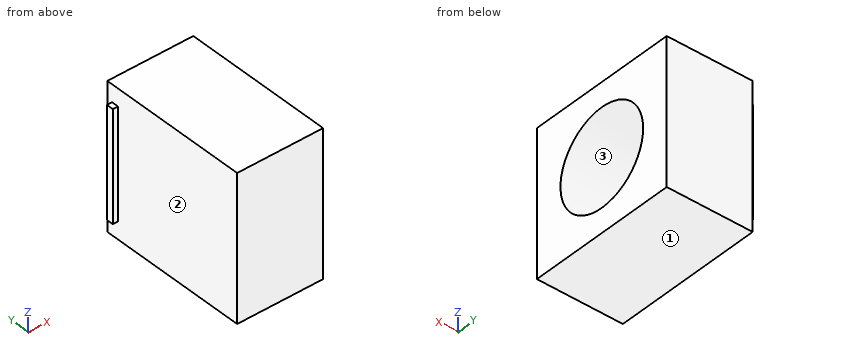
from build123d import *

# Parameters (mm, degrees)
F0_W     = 79.375
F0_H     = 133.35
F1_DEPTH = 139.7
F2_R     = 44.45
F3_DEPTH = 76.2
F4_W     = 6.35
F4_H     = 101.6
F5_DEPTH = 44.45


# Not quite as in the source:
# - a feature names something its author has since deleted; it is built from what else it names


with BuildPart() as f1:
    # F0 (on Front) → F1 (new body)
    with BuildSketch(Plane.XZ):
        Rectangle(F0_W, F0_H)
    extrude(amount=F1_DEPTH)

    # F2 (on face) → F3 (cut)
    with BuildSketch(Plane.YZ.offset(39.6875)):
        with Locations((-69.85, 0)):
            Circle(F2_R)
    extrude(amount=-F3_DEPTH, mode=Mode.SUBTRACT)

    # F4 (on Right) → F5 (join)
    with BuildSketch(Plane.YZ):
        with Locations((-8.2414448261, 0)):
            Rectangle(F4_W, F4_H)
    extrude(amount=-F5_DEPTH)


solid = f1.part
Design review of the part built by this model. Coordinates are the model's own, in mm. Face numbers are marked on the shaded views. Round coordinates to 2 decimals unless told otherwise and drop trailing zeros. Write each loop counter-clockwise with the first axis right and the second up, starting at its lowest first coordinate (ties: lowest second). Pieces come first, ordered by that corner, then holes. Notation, with made-up numbers: (82, -29.5) -> (88, -29.5) arc R5 ccw to (88, -21.5) -> close; hole circle Ø6 at (34, -15.5). An arc over 180 degrees is marked (long way). One line per item, written item: value. Start each with the question number.
Q1. Add section C-C (x = 4.5). Give the boundary of the cut face in (y, z) (3 decimals), then the cut area to 3 significant figures.
Q2. The part is to be moulded in two halves that separate along Z. For the marked faces 1, 2 and 3, say which applies: pulls with the +Z half, pulls with the -Z half, needs draft (parallel to the pull), parting line crosses it, or undercut.
Q3. Add section D-D (y = -92.5). Give the boundary of the cut face in (x, z) (1 decimal).
Q4. To check wall thickness, follow probe 1 along Z at (x, y) = (11.5, -69.85) (3 decimals); probe 2 along X at (y, z) = (-31, -42.5); probe 3 along X at (y, z) = (-71, 34). State the ranges of each line that lie inside material, in increasing order.
Q5. Add section B-B (z = 0). Give the boundary of the cut face in (x, y), then the cut area to 3 significant figures.
Q6. Insertion check: P1, Ø1.5, axis at y = -53.5, z = 24.5, coming from the -X side; P2, Ø3, axis at y = -79, z = 24, coming from the +X side; P3, Ø4, axis at x = -42, y = -7, coming from the +Z side. Each pin has a flat end and moves straight along its axis. Give the tip position at first contact, or say it passes through.
Response:
1. outline: (-139.7, -66.675) -> (0, -66.675) -> (0, 66.675) -> (-139.7, 66.675) -> close; hole circle Ø88.9 at (-69.85, 0)
1. area: 12,400 mm^2
2. face 1: pulls with the -Z half
2. face 2: needs draft
2. face 3: undercut
3. outline: (-39.7, -66.7) -> (39.7, -66.7) -> (39.7, -38.2) -> (-36.5, -38.2) -> (-36.5, 38.2) -> (39.7, 38.2) -> (39.7, 66.7) -> (-39.7, 66.7) -> close
4. probe 1: z = -66.675 to -44.45, 44.45 to 66.675
4. probe 2: x = -39.69 to 39.69
4. probe 3: x = -39.69 to -36.51
5. outline: (-44.45, -11.42) -> (-39.69, -11.42) -> (-39.69, -139.7) -> (39.69, -139.7) -> (39.69, -114.3) -> (-36.51, -114.3) -> (-36.51, -25.4) -> (39.69, -25.4) -> (39.69, 0) -> (-39.69, 0) -> (-39.69, -5.07) -> (-44.45, -5.07) -> close
5. area: 4,340 mm^2
6. P1: stops at x = -39.69
6. P2: stops at x = -36.51
6. P3: stops at z = 50.8
